Input: part model. Units: mm. Frame: model coordinates. Face numbers are marked on the shaded views. A direction names the side the tool comes from. Give positions to 0.01 mm unless a question says otherwise; leave off trailing zeros. Loops run counter-clockwise (first coordinate to the right, second up) from the corner with the lowest first, then second, coordinate; pieces in that order, holes last. Notation, with made-up numbers: M 79,9 L 127,9 A16 ccw 127,16 Z; hole C -23.75,73.5 d11. An arc over 180 degrees is marked long. Answer as a JSON object with one key per item and string values. Group by question number.
1) Draft query along Y for the marked faces 4, 5, 6 and 7. Return one class per face: +Y half, -Y half, draft (parallel to the pull), parting line (faces both ways), or undercut.
2) Section query D-D on z = 5.1. Return loops of the section in (x, y).
3) First-contact query: P1, Ø4, axis at x = 0, y = 15, coming from the +Z side. Flat tip, straight axial feed; report the tip coordinate or a pass-through.
4) Access query for the marked faces 1, 2 and 3. Directions: +Z, -Z, +X, -X, +Y, -Y. A direction counts if a zero-diameter tool reaches every point of the face in a straight line with its end or side. Return the directions, or none.
5) Section query C-C on z = 1.1. Return loops of the section in (x, y), plus the area to 3 significant figures.
6) Ray query, L1, parallel to Y at x = 0, z = 1.5; L2, parallel to Y at x = 0, z = 4; L3, parallel to X at y = -8.5, z = 0.5. Return the intervals inside material, ascending.
7) Section query B-B on x = 0. Return loops of the section in (y, z), plus the area to 3 significant figures.
8) Section query A-A on y = -14. Return loops of the section in (x, z), plus the area to 3 significant figures.
from build123d import *
from build123d.topology import SkipClean

# Parameters (mm, degrees)
SKETCH1_R           = 1.25
BOSS_EXTRUDE1_DEPTH = 3
SKETCH2_R           = 4
SKETCH2_R_2         = 3
BOSS_EXTRUDE2_DEPTH = 3


with BuildPart() as part:
    # Sketch1 → Boss-Extrude1 (new body)
    with BuildSketch(Plane.XY):
        with BuildLine():
            Line((4, 15), (4, -15))
            ThreePointArc((4, -15), (0, -19), (-4, -15))
            Line((-4, -15), (-4, 15))
            ThreePointArc((-4, 15), (0, 19), (4, 15))
        make_face()
        with Locations((0, 15)):
            Circle(SKETCH1_R, mode=Mode.SUBTRACT)
        with BuildLine():
            Line((-2, -5), (-2, -15))
            ThreePointArc((-2, -15), (0, -17), (2, -15))
            Line((2, -15), (2, -5))
            ThreePointArc((2, -5), (0, -3), (-2, -5))
        make_face(mode=Mode.SUBTRACT)
    extrude(amount=BOSS_EXTRUDE1_DEPTH)

    # Sketch2 → Boss-Extrude2 (add)
    with SkipClean():  # the faces are left unmerged after this step: merging them gives an invalid solid
        with BuildSketch(Plane.XY.offset(3)):
            with Locations((0, 15)):
                Circle(SKETCH2_R)
            with Locations((0, 15)):
                Circle(SKETCH2_R_2, mode=Mode.SUBTRACT)
        extrude(amount=BOSS_EXTRUDE2_DEPTH)
    add(part.part.scale(1), mode=Mode.REPLACE)  # the faces are merged on a copy


solid = part.part
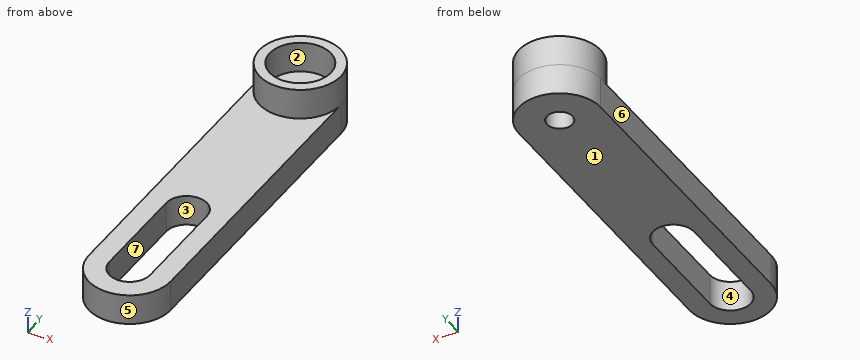
Output:
{
 "1": {"face 4": "undercut", "face 5": "-Y half", "face 6": "draft", "face 7": "undercut"},
 "2": {"outline": "C 0,15 d8; hole C 0,15 d6"},
 "3": {"P1": "stops at z = 3"},
 "4": {"face 1": "-Z, +X, -X, +Y, -Y", "face 2": "+Z", "face 3": "+Z, -Z"},
 "5": {"outline": "M -4,-15 A4 ccw 4,-15 L 4,15 A4 ccw -4,15 Z; hole M -2,-15 A2 ccw 2,-15 L 2,-5 A2 ccw -2,-5 Z; hole C 0,15 d2.5", "area": "233 mm^2"},
 "6": {"L1": "y = -19 to -17, -3 to 13.75, 16.25 to 19", "L2": "y = 11 to 12, 18 to 19", "L3": "x = -4 to -2, 2 to 4"},
 "7": {"outline": "M -19,0 L -17,0 L -17,3 L -19,3 Z; M -3,0 L 13.75,0 L 13.75,3 L 12,3 L 12,6 L 11,6 L 11,3 L -3,3 Z; M 16.25,0 L 19,0 L 19,6 L 18,6 L 18,3 L 16.25,3 Z", "area": "70.5 mm^2"},
 "8": {"outline": "M -4,0 L -2,0 L -2,3 L -4,3 Z; M 2,0 L 4,0 L 4,3 L 2,3 Z", "area": "12.0 mm^2"}
}
